Work out the finished part from the listing and answer in its coordinate system (mm). A direction names the side the tool comes from. Round coordinates to 2 decimals unless told otherwise and drop trailing zeros. Order: outer loops, then holes, each group sorted by start corner. A loop starts at its lowest first (then second) coordinate and runs counter-clockwise, first axis right, second up. Notation, with made-up numbers: (25.25, -21) -> (60.25, -21) arc R24 ccw to (60.25, -2) -> close; hole circle Ø9 at (80, -30). An arc over 180 degrees is marked (long way). Use a Markdown table: item, result. Add a question column.
Item 1: A cutting plane is placed at C-C, the plane z = 0. Determine the outline of the cut face in (x, y) (3 decimals).
Item 2: Flat-ended cylindrical pins translate along their axes: P1, Ø1, axis at x = 1, z = -0.5, coming from the +Y side; P2, Ø2, axis at x = 3, y = -1.5, coming from the -Z side. Find the tip coordinate at first contact, or state that the pin passes through.
Item 3: A cutting plane is placed at D-D, the plane x = 1. Determine the outline of the cut face in (y, z) (3 decimals).
Item 4: Find the intervals of material crossed by L1, parallel to Y at x = 2.5, z = -1.25; L2, parallel to Z at x = 2, y = -1.35; L3, parallel to Y at x = 7.25, z = -1.15, in increasing order. Write a range as [from, to].
Item 5: A cutting plane is placed at B-B, the plane x = 2. Determine the outline of the cut face in (y, z), plus the area to 3 significant figures.
Item 6: A cutting plane is placed at A-A, the plane y = 0. Determine the outline of the cut face in (x, z) (3 decimals).
Item 7: A tool of negligible diameter and unlimited length cuts with its end or side. For faces 1 (the cylindrical face through (4.79, -1.5, -0.07)), 2 (the cylindrical face through (0.205, -0.596, 2.685)), 3 (the flat face through (0.83, 0, 0)), from which of +Z, -Z, +X, -X, +Y, -Y can it reach the whole face along a straight path? Write none if from no direction.
Autodesk Inventor part; units mm, degrees
ref_plane "YZ Plane" through (0, 0, 0) normal (1, 0, 0) x (0, 1, 0)
ref_plane "XZ Plane" through (0, 0, 0) normal (0, 1, 0) x (-1, 0, 0)
ref_plane "XY Plane" through (0, 0, 0) normal (0, 0, 1) x (1, 0, 0)
sketch "Sketch1" plane through (0, 0, 0) normal (0, 0, 1) x (1, 0, 0)
  line L0 (0, 0) -> (8, 0)
  line L1 (8, 0) -> (8, 1.5)
  line L2 (8, 1.5) -> (2.35, 1.5)
  line L3 (2.35, 1.5) -> (2.15, 1.5)
  line L4 (2.15, 1.5) -> (1.67, 1.5)
  line L5 (1.65, 1.515) -> (1.65, 1.515)
  line L6 (1.65, 1.515) -> (0.415, 2.75)
  line L7 (0.415, 2.75) -> (0, 2.75)
  line L8 (0, 2.75) -> (0, 0)
  line L9 (1.65, 1.515) -> (1.65, 1.52)
  arc A0 (1.65, 1.52) -> (1.67, 1.5) centre (1.67, 1.52) ccw
  dimension "d17" = 8
  dimension "d18" = 0.415
  dimension "d19" = 1.65
  dimension "d20" = 0
  dimension "d21" = 5.5
  dimension "d22" = 3
  dimension "d23" = 3
  dimension "d25" = 45
  dimension "d26" = 0.2
  dimension "d28" = 0.02
  dimension "d29" = 5.65
  dimension "d30" = 0.02
  dimension "d52" = 0.7
revolve "Revolution1" add sketch "Sketch1" angle 360 about axis through (0, 0, 0) along (1, 0, 0)
thread "Thread1"
sketch "Sketch2" plane through (0, 0, 0) normal (-1, 0, 0) x (0, 0, 1)
  circle A0 centre (0, 0) radius 1.4 construction
  circle A1 centre (0, 0) radius 0.98 construction
  line L0 (0, 0) -> (0.8487, 0.49)
  line L1 (0, 0) -> (0.98, 0) construction
  line L2 (0, 0) -> (0.8487, -0.49)
  line L3 (0, 0) -> (0.98, 0) construction
  line L4 (0.8487, 0.49) -> (1.4, 0)
  line L5 (1.4, 0) -> (0.8487, -0.49)
  dimension "d34" = 2.8
  dimension "d35" = 1.96
  dimension "d39" = 30
  dimension "d40" = 330
extrude "Extrusion1" cut sketch "Sketch2" against normal blind 0.83
pattern_circular "Circular Pattern1" count 6 over 360 about axis through (-10, 0, 0) along (1, 0, 0) of "Extrusion1"
fillet "Fillet1" radius 0.3 12 edges at (0.415, 0.49, 0.8487) (0.415, 0, 1.4) (0.415, -0.49, 0.8487) (0.415, -0.98, 0) (0.415, -1.2124, 0.7) (0.415, -1.2124, -0.7) (0.415, -0.49, -0.8487) (0.415, 0, -1.4) (0.415, 0.49, -0.8487) (0.415, 1.2124, -0.7) (0.415, 0.98, 0) (0.415, 1.2124, 0.7)
equation "\"d32\" = b"
equation "\"d34\" = A_"
equation "\"d35\" = 0.7 * A_"
equation "\"d43\" = t"
equation "\"d48\" = v"
equation "\"d17\" = l_"
equation "\"d18\" = 0.5 * t"
equation "\"d19\" = k"
equation "\"d21\" = dk"
equation "\"d22\" = d"
equation "\"d23\" = ds_"
equation "\"d25\" = 0.5 * headAngle"
equation "\"d26\" = x"
equation "\"d28\" = r"
equation "\"d29\" = b"
properties part number "Šroub se zápustnou hlavou a šestiramennou drážkou ISO 14581 - M3x8-4.8" material "Ocel, měkká"
Reported:
| question | item | result |
|---|---|---|
| 1 | outline | (0, -2.75) -> (0.415, -2.75) -> (1.65, -1.515) arc R0.02 cw to (1.67, -1.5) -> (8, -1.5) -> (8, 1.5) -> (1.67, 1.5) arc R0.02 cw to (1.651, 1.515) -> (0.415, 2.75) -> (0, 2.75) -> (0, 0.996) -> (0.83, 0.996) -> (0.83, -0.996) -> (0, -0.996) -> close |
| 2 | P1 | y = 2.63 |
| 2 | P2 | z = -1.41 |
| 3 | outline | circle Ø4.33 at (0, 0) |
| 4 | L1 | [-0.83, 0.83] |
| 4 | L2 | [-0.65, 0.65] |
| 4 | L3 | [-0.96, 0.96] |
| 5 | outline | circle Ø3 at (0, 0) |
| 5 | area | 7.07 mm² |
| 6 | outline | (0, -2.75) -> (0.415, -2.75) -> (1.65, -1.515) arc R0.02 cw to (1.67, -1.5) -> (8, -1.5) -> (8, 1.5) -> (1.67, 1.5) arc R0.02 cw to (1.651, 1.515) -> (0.415, 2.75) -> (0, 2.75) -> (0, 1.248) -> (0.83, 1.248) -> (0.83, -1.248) -> (0, -1.248) -> close |
| 7 | face 1 | +X |
| 7 | face 2 | +X, -X |
| 7 | face 3 | -X |
